from build123d import *


with BuildPart() as f1:
    # F0 (on Front) → F1 (revolve)
    with BuildSketch(Plane.XZ):
        with BuildLine():
            Line((-13.495519, -19.783843), (31.504481, -19.783843))
            Line((31.504481, -19.783843), (31.504481, -1.783843))
            ThreePointArc((31.504481, -1.783843), (30.918695, -0.369629), (29.504481, 0.216157))
            Line((29.504481, 0.216157), (24.837814, 0.216157))
            ThreePointArc((24.837814, 0.216157), (22.064313, 1.055906), (20.22243, 3.29308))
            Line((20.22243, 3.29308), (9.773712, 28.370003))
            ThreePointArc((9.773712, 28.370003), (8.668582, 29.712308), (7.004481, 30.216157))
            Line((7.004481, 30.216157), (-13.495519, 30.216157))
            Line((-13.495519, 30.216157), (-13.495519, -19.783843))
        make_face()
    revolve(axis=Axis((-13.495519, 0, 5.240102), (0, 0, -1)))


solid = f1.part
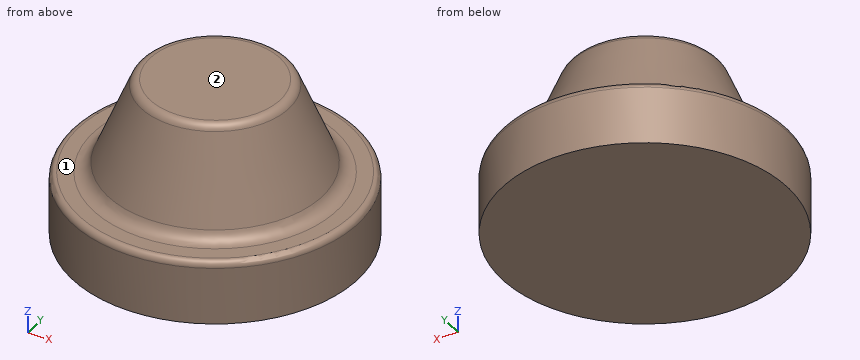
Could you check a few things on this model? Use its own coordinates, in mm. Face numbers are marked on the shaded views. A direction names the side the tool comes from. Coordinates: 2 decimals unless noted, no trailing zeros. Order: outer loops, then holes, each group sorted by start corner. A loop starts at its lowest first (then second) coordinate and runs counter-clockwise, first axis right, second up.
Q1. Suppose I cut it at A-A on y = 0. Please give me the cut outline in (x, z), and give its area (3 significant figures).
Q2. Suppose I cut it at B-B on z = -4. Please give me the cut outline in (x, y).
Q3. Suppose I cut it at C-C on z = 17.5. Please give me the cut outline in (x, y), and give its area (3 significant figures).
Q4. Which directions (+Z, -Z, +X, -X, +Y, -Y) give clear straight access to the entire face, cutting with the end or side of a thin tool? Please do the marked faces 1 and 2.
Q5. Please list where these lines run through material, in increasing order: L1, parallel to Z at x = 12, y = -33.5; L2, parallel to Z at x = -12, y = -22; L3, parallel to X at y = 10, z = -14.5.
Q6. Will these pins go through, and if not, where does the flat tip stop? pin 1 (6 mm diameter, centred on x = -19.5, z = -10, fed in from +Y); pin 2 (1.5 mm diameter, centred on x = -12, z = 24.5, fed in from +Y); pin 3 (10 mm diameter, centred on x = -5, y = -31.5, fed in from +Z).
Answer:
1. outline: (-58.5, -19.78) - (31.5, -19.78) - (31.5, -1.78) arc R2 ccw to (29.5, 0.22) - (24.84, 0.22) arc R5 cw to (20.22, 3.29) - (9.77, 28.37) arc R3 ccw to (7, 30.22) - (-34, 30.22) arc R3 ccw to (-36.76, 28.37) - (-47.21, 3.29) arc R5 cw to (-51.83, 0.22) - (-56.5, 0.22) arc R2 ccw to (-58.5, -1.78) - close
1. area: 3,530 mm2
2. outline: circle Ø90 at (-13.5, 0)
3. outline: circle Ø55.6 at (-13.5, 0)
3. area: 2,430 mm2
4. face 1: +Z
4. face 2: +Z, +X, -X, +Y, -Y
5. L1: z = -19.78 to 0.22
5. L2: z = -19.78 to 29.78
5. L3: x = -57.37 to 30.38
6. pin 1: stops at y = 44.9
6. pin 2: stops at y = 25.15
6. pin 3: stops at z = 17.91
